Source: CAD feature listing. Evaluate the final solid. Frame: model axes, mm. Face numbers are marked on the shaded views. A direction names the side the tool comes from. Round coordinates to 2 decimals unless told otherwise and drop trailing zeros. Write each loop counter-clockwise with the first axis right and the second up, starting at its lowest first coordinate (ties: lowest second). Pieces come first, ordered by that corner, then holes. Notation, with made-up numbers: M -37.5,-3.5 L -1.5,-3.5 A17 ccw -1.5,20.5 Z; hole C 82.5,51.5 d11. An arc over 180 degrees is marked long. Answer in a Markdown table with one row per item.
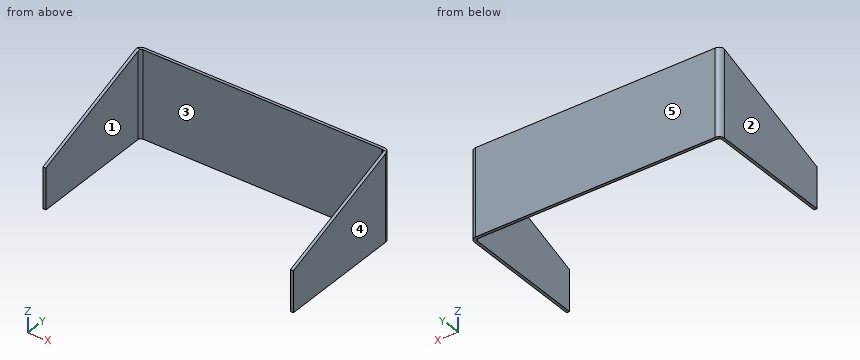
from build123d import *

# Parameters (mm, degrees)
F1_DEPTH = 101.6
F3_DEPTH = 292.101
F4_R     = 3.175
F5_R     = 6.35


with BuildPart() as f1:
    # F0 (on Top) → F1 (new body)
    with BuildSketch(Plane.XY):
        Polygon((0, 152.4), (0, 0), (3.429, 0), (3.429, 148.971), (288.671, 148.971), (288.671, 0), (292.1, 0), (292.1, 152.4), align=None)
    extrude(amount=F1_DEPTH)

    # F2 (on face) → F3 (cut, through all)
    with BuildSketch(Plane.YZ.offset(292.1)):
        Polygon((0, 101.6), (0, 47.625), (148.295094, 101.6), align=None)
    extrude(amount=-F3_DEPTH, mode=Mode.SUBTRACT)

    # F4
    f4_edges = [f1.edges().sort_by_distance(p)[0] for p in [
        (288.671, 148.971, 50.8),
        (3.429, 148.971, 50.8),
    ]]
    fillet(f4_edges, radius=F4_R)

    # F5
    f5_edges = [f1.edges().sort_by_distance(p)[0] for p in [
        (0, 152.4, 50.8),
        (292.1, 152.4, 50.8),
    ]]
    fillet(f5_edges, radius=F5_R)


solid = f1.part
Q1. Access query for the marked faces 1 and 2. Directions: +Z, -Z, +X, -X, +Y, -Y. A direction counts if a zero-diameter tool reaches every point of the face in a straight line with its end or side. Return the directions, or none.
Solutions:
| item | result |
|---|---|
| face 1 | +Z, -Z, -Y |
| face 2 | +Z, -Z, -X, +Y, -Y |
Q2. Material intervals for probe 1 along X at (y, z) = (124.5, 41); probe 2 along Y at (x, z) = (215, 92.5), sorted ascending.
Solutions:
| item | result |
|---|---|
| probe 1 | x = 0 to 3.43, 288.67 to 292.1 |
| probe 2 | y = 148.97 to 152.4 |
Q3. Contact query for a flat-ended pin moving along its axis: pin 1 Ø3 at (x, z) = (53, 46) entering from -Y. Output: stop coordinate, or through.
Solutions:
| item | result |
|---|---|
| pin 1 | stops at y = 148.97 |
Q4. Section A-A (y = 36.5). Return loops of the section in (x, z).
Solutions:
| item | result |
|---|---|
| outline | M 0,0 L 3.43,0 L 3.43,60.91 L 0,60.91 Z; M 288.67,0 L 292.1,0 L 292.1,60.91 L 288.67,60.91 Z |
Q5. Section B-B (z = 42). Return loops of the section in (x, y) (3 decimals), and give its area (3 significant figures).
Solutions:
| item | result |
|---|---|
| outline | M 0,0 L 3.429,0 L 3.429,145.796 A3.175 cw 6.604,148.971 L 285.496,148.971 A3.175 cw 288.671,145.796 L 288.671,0 L 292.1,0 L 292.1,146.05 A6.35 ccw 285.75,152.4 L 6.35,152.4 A6.35 ccw 0,146.05 Z |
| area | 2,010 mm2 |
Q6. Pull-direction query (X, two-part tool) for the marked faces 3, 4 and 5; classes: pulls with the +X half, pulls with the -X half, needs draft (parallel to the pull), parting line crosses it, or undercut.
Solutions:
| item | result |
|---|---|
| face 3 | undercut |
| face 4 | pulls with the +X half |
| face 5 | needs draft |
Q7. Section C-C (y = 82.5). Return loops of the section in (x, z), and give its area (3 significant figures).
Solutions:
| item | result |
|---|---|
| outline | M 0,0 L 3.43,0 L 3.43,77.65 L 0,77.65 Z; M 288.67,0 L 292.1,0 L 292.1,77.65 L 288.67,77.65 Z |
| area | 533 mm2 |
Q8. Section D-D (x = 155.5). Return loops of the section in (y, z).
Solutions:
| item | result |
|---|---|
| outline | M 148.97,0 L 152.4,0 L 152.4,101.6 L 148.97,101.6 Z |
